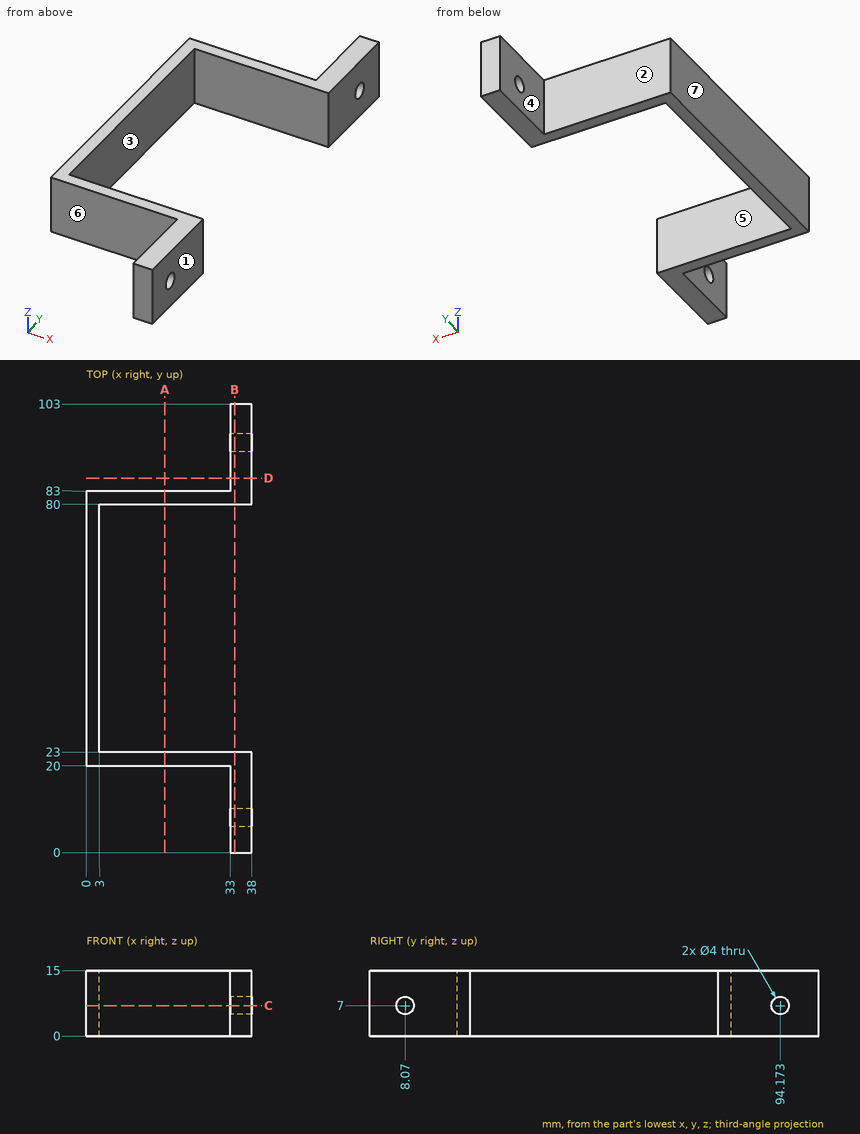
Answer from the drawing. Dimensions are ordinates in mm from the lowest x, y and z of the part. A direction names the side the tool comes from. Round coordinates to 2 decimals unless told otherwise and drop trailing zeros. Order: outer loops, then holes, each group sorted by start corner. A loop starts at its lowest first (then second) coordinate and runs counter-clockwise, first axis right, second up. Notation, with made-up numbers: (63, 23) -> (102, 23) arc R10 cw to (102, 41) -> close; hole circle Ø1 at (23.25, 30). An arc over 180 degrees is marked (long way). Answer as CSV lines item,"result".
Q1. Given pin 1 (4.5 mm diameter, centred on x = 12, z = 6, fed in from +Y); pin 2 (5 mm diameter, centred on y = 32, z = 5.5, fed in from -X); pin 3 (7.5 mm diameter, centred on y = 97.5, z = 7, fed in from -X); pin 4 (7.5 mm diameter, centred on y = 47, z = 5, fed in from +X), each flat-ended and moving along its own axis, determine where each tip first touches the part or whether it passes through.
Computed values:
pin 1,"stops at y = 83"
pin 2,"stops at x = 0"
pin 3,"stops at x = 33"
pin 4,"stops at x = 3"
Q2. Consider line 1 (Y direction, x = 26.5, z = 1); line 2 (Y direction, x = 36.5, z = 2.5); line 3 (X direction, y = 98, z = 11.5). Determine where each line is inside the solid, lowest interval first. Write a range as from..to.
Computed values:
line 1,"y = 20..23, 80..83"
line 2,"y = 0..23, 80..103"
line 3,"x = 33..38"
Q3. A cutting plane is placed at C-C on z = 7. Determine the outline of the cut face in (x, y).
Computed values:
outline,"(0, 20) -> (33, 20) -> (33, 10.07) -> (38, 10.07) -> (38, 23) -> (3, 23) -> (3, 80) -> (38, 80) -> (38, 92.17) -> (33, 92.17) -> (33, 83) -> (0, 83) -> close; (33, 0) -> (38, 0) -> (38, 6.07) -> (33, 6.07) -> close; (33, 96.17) -> (38, 96.17) -> (38, 103) -> (33, 103) -> close"
Q4. A cutting plane is placed at B-B on x = 34. Determine the outline of the cut face in (y, z), plus the area to 3 significant figures.
Computed values:
outline,"(0, 0) -> (23, 0) -> (23, 15) -> (0, 15) -> close; (80, 0) -> (103, 0) -> (103, 15) -> (80, 15) -> close; hole circle Ø4 at (8.07, 7); hole circle Ø4 at (94.17, 7)"
area,"665 mm^2"
Q5. Which of the six approach directions +Z, -Z, +X, -X, +Y, -Y give full straight-line access (tool end or side, diameter ignored) to the marked faces 4, 5, 6 and 7?
Computed values:
face 4,"+Z, -Z, -X, +Y"
face 5,"+Z, -Z, +X"
face 6,"+Z, -Z, -X, -Y"
face 7,"+Z, -Z, -X, +Y, -Y"
Q6. For a pull along Y with two mould halves and no side action, classify the marked faces 1, 2 and 3 as +Y half, -Y half, draft (parallel to the pull), parting line (faces both ways), or undercut.
Computed values:
face 1,"draft"
face 2,"+Y half"
face 3,"undercut"
Q7. A cutting plane is placed at D-D on y = 86. Determine the outline of the cut face in (x, z), plus the area to 3 significant figures.
Computed values:
outline,"(33, 0) -> (38, 0) -> (38, 15) -> (33, 15) -> close"
area,"75.0 mm^2"
Q8. A cutting plane is placed at A-A on x = 18. Determine the outline of the cut face in (y, z).
Computed values:
outline,"(20, 0) -> (23, 0) -> (23, 15) -> (20, 15) -> close; (80, 0) -> (83, 0) -> (83, 15) -> (80, 15) -> close"
